Autodesk Fusion 360 part; units mm, degrees
sketch "Esquisse1" plane through (0, 0, 0) normal (0, 0, 1) x (1, 0, 0)
  line L0 (27.5, -52.5) -> (-27.5, -52.5)
  line L1 (-52.5, -27.5) -> (-52.5, 27.5)
  line L2 (-27.5, 52.5) -> (27.5, 52.5)
  line L3 (52.5, 27.5) -> (52.5, -27.5)
  circle A0 centre (0, 0) radius 52.5
  line L4 (40, -40) -> (-40, 40) construction
  line L5 (-40, -40) -> (40, 40) construction
  circle A1 centre (-40, -40) radius 1.25
  circle A2 centre (40, -40) radius 1.25
  circle A3 centre (-40, 40) radius 1.25
  circle A4 centre (40, 40) radius 1.25
  arc A5 (-52.5, -27.5) -> (-27.5, -52.5) centre (-27.5, -27.5) ccw
  arc A6 (27.5, -52.5) -> (52.5, -27.5) centre (27.5, -27.5) ccw
  arc A7 (52.5, 27.5) -> (27.5, 52.5) centre (27.5, 27.5) ccw
  arc A8 (-27.5, 52.5) -> (-52.5, 27.5) centre (-27.5, 27.5) ccw
  dimension "d3" = 105
  dimension "d40" = 2.5
  dimension "d41" = 2.5
  dimension "d42" = 2.5
  dimension "d43" = 2.5
extrude "Extrusion1" add sketch "Esquisse1" along normal blind 5
sketch "Esquisse2" plane through (0, 0, 5) normal (0, 0, 1) x (-1, 0, 0)
  line L0 (-27.5, -52.5) -> (27.5, -52.5)
  line L1 (52.5, -27.5) -> (52.5, 27.5)
  line L2 (27.5, 52.5) -> (-27.5, 52.5)
  line L3 (-52.5, 27.5) -> (-52.5, -27.5)
  circle A0 centre (0, 0) radius 48
  arc A1 (-52.5, -27.5) -> (-27.5, -52.5) centre (-27.5, -27.5) ccw
  arc A2 (27.5, -52.5) -> (52.5, -27.5) centre (27.5, -27.5) ccw
  arc A3 (52.5, 27.5) -> (27.5, 52.5) centre (27.5, 27.5) ccw
  arc A4 (-27.5, 52.5) -> (-52.5, 27.5) centre (-27.5, 27.5) ccw
  dimension "d16" = 96
extrude "Extrusion2" add sketch "Esquisse2" along normal blind 25 draft -18 contours A0
hole "Perçage2" at (0, 0, 0) direction (0, 0, 1) diameter 80 depth 60 tip angle 180
sketch "Esquisse5" plane through (0, 0, 0) normal (1, 0, 0) x (0, 1, 0)
sketch "Esquisse6" plane through (0, 0, 0) normal (0, 0, 1) x (1, 0, 0)
  circle A0 centre (0, 0) radius 40
  dimension "d28" = 80
extrude "Extrusion4" add sketch "Esquisse6" along normal blind 60
hole "Perçage3" at (0, 0, 0) direction (0, 0, 1) diameter 80 depth 5 tip angle 118
extrude "Extrusion6" cut sketch "Esquisse1" along normal blind 5 contours A1 | A2 | A3 | A4
Work out the finished part from the listing and answer in its coordinate system (mm). A direction names the side the tool comes from. Round coordinates to 2 decimals unless told otherwise and drop trailing zeros. Write each loop counter-clockwise with the first axis right and the second up, starting at its lowest first coordinate (ties: lowest second). Pieces come first, ordered by that corner, then holes.
1) The mould has two halves that part along X. Classify faces 1 (the cylindrical face through (-41.25, 39.95, 2.46)), 2 (the cylindrical face through (-8.67, 39.05, 44.6)), 3 (the flat face through (0, -52.5, 2)): pulls with the +X half, pulls with the -X half, needs draft (parallel to the pull), parting line crosses it, or undercut.
2) A tool of negligible diameter and unlimited length cuts with its end or side. For faces 4 (the cylindrical face through (39.05, -8.67, 2.54)), 5 (the flat face through (-12, 47, 5)), 6 (the cylindrical face through (-41.25, -40.05, 2.46)), from which of +Z, -Z, +X, -X, +Y, -Y can it reach the whole face along a straight path? Write none if from no direction.
3) A cutting plane is placed at A-A (z = 19.5). Give the vertices of the cut face in (x, y).
4) Given pin 1 Ø2 at (x, y) = (40, 40) entering from +Z (1 decimal); pin 2 Ø8 at (x, z) = (-20.5, 9.5) entering from +Y; pin 3 Ø6 at (y, z) = (26, 37) entering from +X; pin 4 Ø12 at (x, z) = (15, 49) entering from +Y, each flat-ended and moving along its own axis, determine where each tip first touches the part or whether it passes through.
5) Straight lines are drawn through the part: line 1 (Y direction, x = -1.5, z = 4.5); line 2 (Z direction, x = -23.5, y = 43.5). For each, find the intervals that lie inside material, in ascending order.
Completed:
1. face 1: undercut
1. face 2: parting line crosses it
1. face 3: needs draft
2. face 4: -Z
2. face 5: +Z
2. face 6: +Z, -Z
3. outline: circle Ø86.58 at (0, 0); hole circle Ø31.74 at (0, 0)
4. pin 1: passes through
4. pin 2: stops at y = 44.05
4. pin 3: stops at x = 32.73
4. pin 4: stops at y = 38.97
5. line 1: y = -52.5 to -39.97, 39.97 to 52.5
5. line 2: z = 0 to 5
